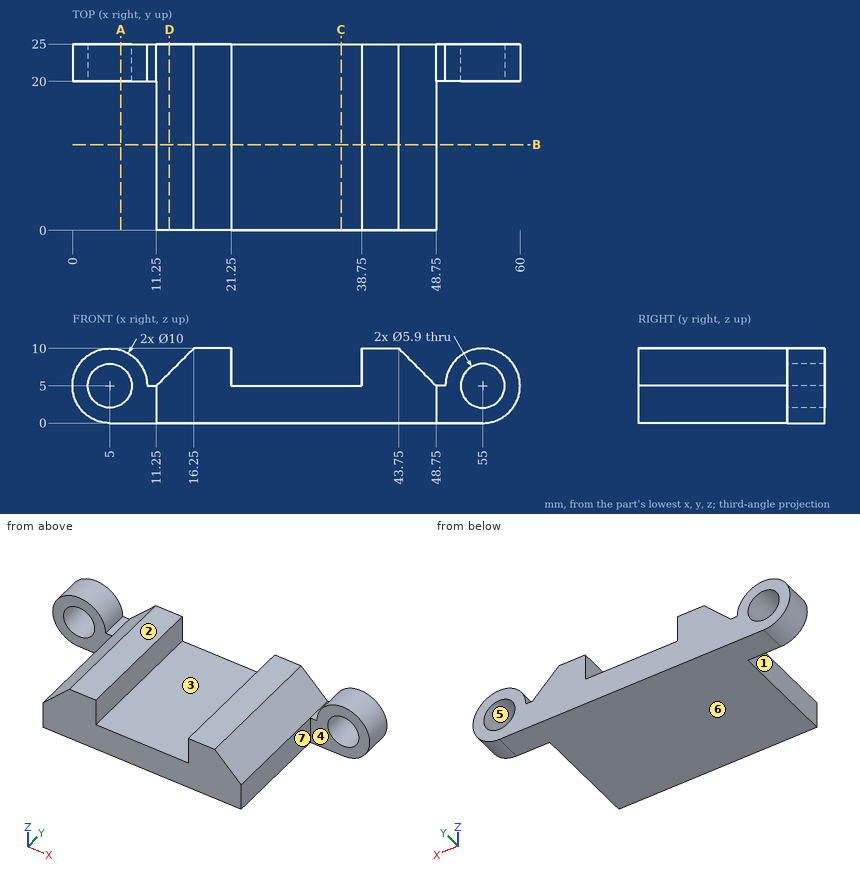
Study the drawing (mm; zero at the part's minimum x, y, z) and answer. A direction names the side the tool comes from. Round coordinates to 2 decimals unless told otherwise and drop trailing zeros. Loops run counter-clockwise (first coordinate to the right, second up) from the corner with the lowest first, then second, coordinate; pieces in that order, holes last.
Q1. Find the intervals of material crossed by line 1 (Z direction, x = 55, y = 22.3); line 2 (X direction, y = 21, z = 6.75); line 3 (X direction, y = 23, z = 6.5), in increasing order.
Q2. Section C-C, the plane x = 36 is taken. Determine the outline of the cut face in (y, z), then the cut area to 3 significant figures.
Q3. For a pull along Z with two mould halves and no side action, classify the marked faces 5, 6 and 7 as released by +Z, released by -Z, zero draft, split by the parting line, or undercut.
Q4. Section A-A, the plane x = 6.5 is taken. Determine the outline of the cut face in (y, z).
Q5. Section D-D, the plane x = 13 is taken. Determine the outline of the cut face in (y, z), then the cut area to 3 significant figures.
Q6. Which of the six approach directions +Z, -Z, +X, -X, +Y, -Y give full straight-line access (tool end or side, diameter ignored) to the marked faces 1, 2, 3 and 4?
Q7. Section B-B, the plane y = 11.5 is taken. Determine the outline of the cut face in (x, z).
Q8. Given pin 1 Ø2.5 at (y, z) = (18, 8) entering from +X; pin 2 Ø3 at (x, z) = (54, 5) entering from -Y; pin 3 Ø5.5 at (y, z) = (5, 2) entering from -X; pin 4 Ø6 at (y, z) = (16.5, 6.5) entering from +X, each flat-ended and moving along its own axis, determine where each tip first touches the part or whether it passes through.
Completed:
1. line 1: z = 0 to 2.05, 7.95 to 10
1. line 2: x = 0.32 to 2.63, 7.37 to 9.68, 13 to 21.25, 38.75 to 47, 50.32 to 52.63, 57.37 to 59.68
1. line 3: x = 0.23 to 2.46, 7.54 to 9.77, 12.75 to 21.25, 38.75 to 47.25, 50.23 to 52.46, 57.54 to 59.77
2. outline: (0, 0) - (25, 0) - (25, 5) - (0, 5) - close
2. area: 125 mm2
3. face 5: undercut
3. face 6: released by -Z
3. face 7: zero draft
4. outline: (20, 0) - (25, 0) - (25, 2.46) - (20, 2.46) - close; (20, 7.54) - (25, 7.54) - (25, 9.77) - (20, 9.77) - close
5. outline: (0, 0) - (25, 0) - (25, 6.75) - (0, 6.75) - close
5. area: 169 mm2
6. face 1: +Z, -Z, -X, -Y
6. face 2: +Z, +X, -X, +Y, -Y
6. face 3: +Z, +Y, -Y
6. face 4: +Z, -Z, +X, -Y
7. outline: (11.25, 0) - (48.75, 0) - (48.75, 5) - (43.75, 10) - (38.75, 10) - (38.75, 5) - (21.25, 5) - (21.25, 10) - (16.25, 10) - (11.25, 5) - close
8. pin 1: stops at x = 47
8. pin 2: passes through
8. pin 3: stops at x = 11.25
8. pin 4: stops at x = 48.75
